Can you work these out from the model? Positions are in its coordinate system, mm. Face numbers are marked on the shaded views. Round coordinates to 2 decimals unless told otherwise and drop trailing zeros. Loops run counter-clockwise (first coordinate to the right, second up) from the corner with the lowest first, then second, coordinate; pieces in that order, holes last. Notation, with made-up numbers: (34.25, 34.5) -> (78.25, 34.5) arc R21 ccw to (78.25, 38.5) -> close; hole circle Ø9 at (37, -29.5). An arc over 180 degrees is marked (long way). Write each question's results on one line, items separated by ' | '.
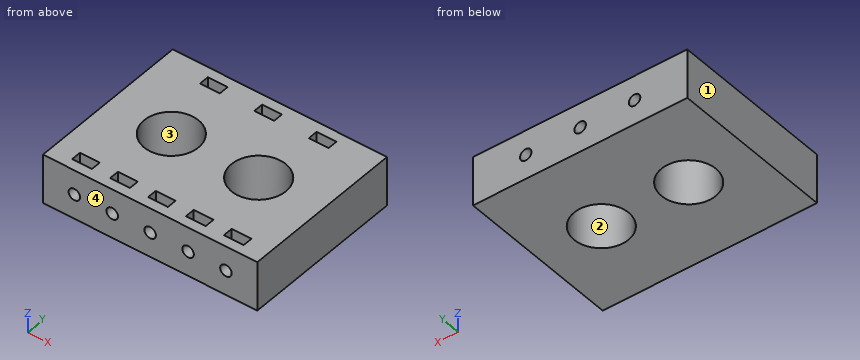
from build123d import *

# Parameters (mm, degrees)
PRISM012_DEPTH            = 3
CYLINDER014_R             = 1.75
CYLINDER014_DEPTH         = 20
BOX014_W                  = 6
BOX014_H                  = 20
BOX014_DEPTH              = 3
FUSION015_PLACEMENT_ANGLE = 180
PRISM013_DEPTH            = 3
CYLINDER015_R             = 1.75
CYLINDER015_DEPTH         = 20
BOX015_W                  = 6
BOX015_H                  = 20
BOX015_DEPTH              = 3
FUSION016_PLACEMENT_ANGLE = 180
PRISM014_DEPTH            = 3
CYLINDER016_R             = 1.75
CYLINDER016_DEPTH         = 20
BOX016_W                  = 6
BOX016_H                  = 20
BOX016_DEPTH              = 3
FUSION017_PLACEMENT_ANGLE = 180
PRISM008_DEPTH            = 3
CYLINDER010_R             = 1.75
CYLINDER010_DEPTH         = 20
BOX010_W                  = 6
BOX010_H                  = 20
BOX010_DEPTH              = 3
PRISM009_DEPTH            = 3
CYLINDER011_R             = 1.75
CYLINDER011_DEPTH         = 20
BOX011_W                  = 6
BOX011_H                  = 20
BOX011_DEPTH              = 3
PRISM010_DEPTH            = 3
CYLINDER012_R             = 1.75
CYLINDER012_DEPTH         = 20
BOX012_W                  = 6
BOX012_H                  = 20
BOX012_DEPTH              = 3
PRISM007_DEPTH            = 3
CYLINDER009_R             = 1.75
CYLINDER009_DEPTH         = 20
BOX009_W                  = 6
BOX009_H                  = 20
BOX009_DEPTH              = 3
PRISM011_DEPTH            = 3
CYLINDER013_R             = 1.75
CYLINDER013_DEPTH         = 20
BOX013_W                  = 6
BOX013_H                  = 20
BOX013_DEPTH              = 3
CYLINDER001_R             = 8.25
CYLINDER001_DEPTH         = 20
CYLINDER_R                = 8.25
CYLINDER_DEPTH            = 20
FUSION_PITCH_ANGLE        = -90
FUSION_PLACEMENT_ANGLE    = 90
BOX_W                     = 65
BOX_H                     = 15
BOX_DEPTH                 = 50
CUT002_PLACEMENT_ANGLE    = 90


with BuildPart() as prisma012:
    # Prism012 → Prism012 (new body)
    with BuildSketch(Plane(origin=(34, 7.5, 3), x_dir=(0, 1, 0), z_dir=(0, 0, 1))):
        Polygon((3.25, 0), (1.625, 2.814583), (-1.625, 2.814583), (-3.25, 0), (-1.625, -2.814583), (1.625, -2.814583), align=None)
    extrude(amount=PRISM012_DEPTH)


with BuildPart() as cilindro014:
    # Cylinder014 → Cylinder014 (new body)
    with BuildSketch(Plane(origin=(34, 7.5, -1), x_dir=(1, 0, 0), z_dir=(0, 0, 1))):
        Circle(CYLINDER014_R)
    extrude(amount=CYLINDER014_DEPTH)


with BuildPart() as fusion015:
    # Box014 → Box014 (new body)
    with BuildSketch(Plane(origin=(31, 9, 3), x_dir=(1, 0, 0), z_dir=(0, 0, 1))):
        with Locations((3, 10)):
            Rectangle(BOX014_W, BOX014_H)
    extrude(amount=BOX014_DEPTH)

    # Fusion015: union Prisma012, Cilindro014
    add(prisma012.part)
    add(cilindro014.part)


with BuildPart() as fusion015_1:
    # Fusion015 placement: moved
    add(fusion015.part.moved(Location((44, 0, 9))).rotate(Axis((44, 0, 9), (0, 1, 0)), FUSION015_PLACEMENT_ANGLE))


with BuildPart() as prisma013:
    # Prism013 → Prism013 (new body)
    with BuildSketch(Plane(origin=(34, 7.5, 3), x_dir=(0, 1, 0), z_dir=(0, 0, 1))):
        Polygon((3.25, 0), (1.625, 2.814583), (-1.625, 2.814583), (-3.25, 0), (-1.625, -2.814583), (1.625, -2.814583), align=None)
    extrude(amount=PRISM013_DEPTH)


with BuildPart() as cilindro015:
    # Cylinder015 → Cylinder015 (new body)
    with BuildSketch(Plane(origin=(34, 7.5, -1), x_dir=(1, 0, 0), z_dir=(0, 0, 1))):
        Circle(CYLINDER015_R)
    extrude(amount=CYLINDER015_DEPTH)


with BuildPart() as fusion016:
    # Box015 → Box015 (new body)
    with BuildSketch(Plane(origin=(31, 9, 3), x_dir=(1, 0, 0), z_dir=(0, 0, 1))):
        with Locations((3, 10)):
            Rectangle(BOX015_W, BOX015_H)
    extrude(amount=BOX015_DEPTH)

    # Fusion016: union Prisma013, Cilindro015
    add(prisma013.part)
    add(cilindro015.part)


with BuildPart() as fusion016_1:
    # Fusion016 placement: moved
    add(fusion016.part.moved(Location((60.5, 0, 9))).rotate(Axis((60.5, 0, 9), (0, 1, 0)), FUSION016_PLACEMENT_ANGLE))


with BuildPart() as prisma014:
    # Prism014 → Prism014 (new body)
    with BuildSketch(Plane(origin=(34, 7.5, 3), x_dir=(0, 1, 0), z_dir=(0, 0, 1))):
        Polygon((3.25, 0), (1.625, 2.814583), (-1.625, 2.814583), (-3.25, 0), (-1.625, -2.814583), (1.625, -2.814583), align=None)
    extrude(amount=PRISM014_DEPTH)


with BuildPart() as cilindro016:
    # Cylinder016 → Cylinder016 (new body)
    with BuildSketch(Plane(origin=(34, 7.5, -1), x_dir=(1, 0, 0), z_dir=(0, 0, 1))):
        Circle(CYLINDER016_R)
    extrude(amount=CYLINDER016_DEPTH)


with BuildPart() as fusion018:
    # Box016 → Box016 (new body)
    with BuildSketch(Plane(origin=(31, 9, 3), x_dir=(1, 0, 0), z_dir=(0, 0, 1))):
        with Locations((3, 10)):
            Rectangle(BOX016_W, BOX016_H)
    extrude(amount=BOX016_DEPTH)

    # Fusion017: union Prisma014, Cilindro016
    add(prisma014.part)
    add(cilindro016.part)


with BuildPart() as fusion018_1:
    # Fusion017 placement: moved
    add(fusion018.part.moved(Location((77, 0, 9))).rotate(Axis((77, 0, 9), (0, 1, 0)), FUSION017_PLACEMENT_ANGLE))

    # Fusion018: union Fusion015, Fusion016
    add(fusion015_1.part)
    add(fusion016_1.part)


with BuildPart() as fusion018_2:
    # Fusion018 placement: moved
    add(fusion018_1.part.moved(Location((6, 0, 0))))


with BuildPart() as prisma008:
    # Prism008 → Prism008 (new body)
    with BuildSketch(Plane(origin=(34, 7.5, 3), x_dir=(0, 1, 0), z_dir=(0, 0, 1))):
        Polygon((3.25, 0), (1.625, 2.814583), (-1.625, 2.814583), (-3.25, 0), (-1.625, -2.814583), (1.625, -2.814583), align=None)
    extrude(amount=PRISM008_DEPTH)


with BuildPart() as cilindro010:
    # Cylinder010 → Cylinder010 (new body)
    with BuildSketch(Plane(origin=(34, 7.5, -1), x_dir=(1, 0, 0), z_dir=(0, 0, 1))):
        Circle(CYLINDER010_R)
    extrude(amount=CYLINDER010_DEPTH)


with BuildPart() as fusion010:
    # Box010 → Box010 (new body)
    with BuildSketch(Plane(origin=(31, 9, 3), x_dir=(1, 0, 0), z_dir=(0, 0, 1))):
        with Locations((3, 10)):
            Rectangle(BOX010_W, BOX010_H)
    extrude(amount=BOX010_DEPTH)

    # Fusion010: union Prisma008, Cilindro010
    add(prisma008.part)
    add(cilindro010.part)


with BuildPart() as fusion010_1:
    # Fusion010 placement: moved
    add(fusion010.part.moved(Location((-9.5, 0, 41))))


with BuildPart() as prisma009:
    # Prism009 → Prism009 (new body)
    with BuildSketch(Plane(origin=(34, 7.5, 3), x_dir=(0, 1, 0), z_dir=(0, 0, 1))):
        Polygon((3.25, 0), (1.625, 2.814583), (-1.625, 2.814583), (-3.25, 0), (-1.625, -2.814583), (1.625, -2.814583), align=None)
    extrude(amount=PRISM009_DEPTH)


with BuildPart() as cilindro011:
    # Cylinder011 → Cylinder011 (new body)
    with BuildSketch(Plane(origin=(34, 7.5, -1), x_dir=(1, 0, 0), z_dir=(0, 0, 1))):
        Circle(CYLINDER011_R)
    extrude(amount=CYLINDER011_DEPTH)


with BuildPart() as fusion011:
    # Box011 → Box011 (new body)
    with BuildSketch(Plane(origin=(31, 9, 3), x_dir=(1, 0, 0), z_dir=(0, 0, 1))):
        with Locations((3, 10)):
            Rectangle(BOX011_W, BOX011_H)
    extrude(amount=BOX011_DEPTH)

    # Fusion011: union Prisma009, Cilindro011
    add(prisma009.part)
    add(cilindro011.part)


with BuildPart() as fusion011_1:
    # Fusion011 placement: moved
    add(fusion011.part.moved(Location((2, 0, 41))))


with BuildPart() as prisma010:
    # Prism010 → Prism010 (new body)
    with BuildSketch(Plane(origin=(34, 7.5, 3), x_dir=(0, 1, 0), z_dir=(0, 0, 1))):
        Polygon((3.25, 0), (1.625, 2.814583), (-1.625, 2.814583), (-3.25, 0), (-1.625, -2.814583), (1.625, -2.814583), align=None)
    extrude(amount=PRISM010_DEPTH)


with BuildPart() as cilindro012:
    # Cylinder012 → Cylinder012 (new body)
    with BuildSketch(Plane(origin=(34, 7.5, -1), x_dir=(1, 0, 0), z_dir=(0, 0, 1))):
        Circle(CYLINDER012_R)
    extrude(amount=CYLINDER012_DEPTH)


with BuildPart() as fusion012:
    # Box012 → Box012 (new body)
    with BuildSketch(Plane(origin=(31, 9, 3), x_dir=(1, 0, 0), z_dir=(0, 0, 1))):
        with Locations((3, 10)):
            Rectangle(BOX012_W, BOX012_H)
    extrude(amount=BOX012_DEPTH)

    # Fusion012: union Prisma010, Cilindro012
    add(prisma010.part)
    add(cilindro012.part)


with BuildPart() as fusion012_1:
    # Fusion012 placement: moved
    add(fusion012.part.moved(Location((13.5, 0, 41))))


with BuildPart() as prisma007:
    # Prism007 → Prism007 (new body)
    with BuildSketch(Plane(origin=(34, 7.5, 3), x_dir=(0, 1, 0), z_dir=(0, 0, 1))):
        Polygon((3.25, 0), (1.625, 2.814583), (-1.625, 2.814583), (-3.25, 0), (-1.625, -2.814583), (1.625, -2.814583), align=None)
    extrude(amount=PRISM007_DEPTH)


with BuildPart() as cilindro009:
    # Cylinder009 → Cylinder009 (new body)
    with BuildSketch(Plane(origin=(34, 7.5, -1), x_dir=(1, 0, 0), z_dir=(0, 0, 1))):
        Circle(CYLINDER009_R)
    extrude(amount=CYLINDER009_DEPTH)


with BuildPart() as fusion009:
    # Box009 → Box009 (new body)
    with BuildSketch(Plane(origin=(31, 9, 3), x_dir=(1, 0, 0), z_dir=(0, 0, 1))):
        with Locations((3, 10)):
            Rectangle(BOX009_W, BOX009_H)
    extrude(amount=BOX009_DEPTH)

    # Fusion009: union Prisma007, Cilindro009
    add(prisma007.part)
    add(cilindro009.part)


with BuildPart() as fusion009_1:
    # Fusion009 placement: moved
    add(fusion009.part.moved(Location((-21, 0, 41))))


with BuildPart() as prisma011:
    # Prism011 → Prism011 (new body)
    with BuildSketch(Plane(origin=(34, 7.5, 3), x_dir=(0, 1, 0), z_dir=(0, 0, 1))):
        Polygon((3.25, 0), (1.625, 2.814583), (-1.625, 2.814583), (-3.25, 0), (-1.625, -2.814583), (1.625, -2.814583), align=None)
    extrude(amount=PRISM011_DEPTH)


with BuildPart() as cilindro013:
    # Cylinder013 → Cylinder013 (new body)
    with BuildSketch(Plane(origin=(34, 7.5, -1), x_dir=(1, 0, 0), z_dir=(0, 0, 1))):
        Circle(CYLINDER013_R)
    extrude(amount=CYLINDER013_DEPTH)


with BuildPart() as fusion014:
    # Box013 → Box013 (new body)
    with BuildSketch(Plane(origin=(31, 9, 3), x_dir=(1, 0, 0), z_dir=(0, 0, 1))):
        with Locations((3, 10)):
            Rectangle(BOX013_W, BOX013_H)
    extrude(amount=BOX013_DEPTH)

    # Fusion013: union Prisma011, Cilindro013
    add(prisma011.part)
    add(cilindro013.part)


with BuildPart() as fusion014_1:
    # Fusion013 placement: moved
    add(fusion014.part.moved(Location((25, 0, 41))))

    # Fusion014: union Fusion010, Fusion011, Fusion012, Fusion009
    add(fusion010_1.part)
    add(fusion011_1.part)
    add(fusion012_1.part)
    add(fusion009_1.part)


with BuildPart() as fusion014_2:
    # Fusion014 placement: moved
    add(fusion014_1.part.moved(Location((-3.5, 0, 0))))


with BuildPart() as cilindro001:
    # Cylinder001 → Cylinder001 (new body)
    with BuildSketch(Plane(origin=(10, 36.5, 0), x_dir=(1, 0, 0), z_dir=(0, 0, 1))):
        Circle(CYLINDER001_R)
    extrude(amount=CYLINDER001_DEPTH)


with BuildPart() as fusion:
    # Cylinder → Cylinder (new body)
    with BuildSketch(Plane(origin=(10, 10, 0), x_dir=(1, 0, 0), z_dir=(0, 0, 1))):
        Circle(CYLINDER_R)
    extrude(amount=CYLINDER_DEPTH)

    # Fusion: union Cilindro001
    add(cilindro001.part)


with BuildPart() as fusion_1:
    # Fusion pitch: moved
    add(fusion.part.rotate(Axis((0, 0, 0), (0, 1, 0)), FUSION_PITCH_ANGLE))


with BuildPart() as fusion_2:
    # Fusion placement: moved
    add(fusion_1.part.moved(Location((55.75, 17, 15))).rotate(Axis((55.75, 17, 15), (0, 0, 1)), FUSION_PLACEMENT_ANGLE))


with BuildPart() as cut002:
    # Box → Box (new body)
    with BuildSketch(Plane.XY):
        with Locations((32.5, 7.5)):
            Rectangle(BOX_W, BOX_H)
    extrude(amount=BOX_DEPTH)

    # Cut: cut Fusion
    add(fusion_2.part, mode=Mode.SUBTRACT)

    # Cut001: cut Fusion014
    add(fusion014_2.part, mode=Mode.SUBTRACT)

    # Cut002: cut Fusion018
    add(fusion018_2.part, mode=Mode.SUBTRACT)


with BuildPart() as cut002_1:
    # Cut002 placement: moved
    add(cut002.part.rotate(Axis((0, 0, 0), (1, 0, 0)), CUT002_PLACEMENT_ANGLE))


solid = cut002_1.part
1. Please list where these lines run through material, in increasing order: line 1 (X direction, y = -25, z = 7.5); line 2 (X direction, y = -17.5, z = 9.5); line 3 (Y direction, x = 18.5, z = 9.5). Write a range as from..to.
Final values:
line 1: 0..11, 27.5..37.5, 54..65 | line 2: 0..15.81, 22.69..42.31, 49.19..65 | line 3: -50..-47, -44..-33.22, -16.78..-6, -3..0
2. If we section it at C-C (y = -8): List the corners of the cut face in (x, z) for me.
Final values:
outline: (0, 0) -> (65, 0) -> (65, 15) -> (0, 15) -> close; hole circle Ø3.5 at (16, 7.5); hole circle Ø3.5 at (32.5, 7.5); hole circle Ø3.5 at (49, 7.5)
3. If we section it at D-D (z = 12.5): State how many separate pieces and enclosed holes the cut face has, then the cut area to 3 significant figures.
Final values:
separate pieces: 1 | enclosed holes: 10 | area: 2,680 mm2
4. We'd pull the mould along X, two halves only. Please class the marked faces 1, 2, 3 and 4: pulls with the +X half, pulls with the -X half, needs draft (parallel to the pull), parting line crosses it, or undercut.
Final values:
face 1: pulls with the -X half | face 2: undercut | face 3: undercut | face 4: needs draft
5. If we section it at B-B (z = 3.5): List the corners of the cut face in (x, y) for me.
Final values:
outline: (0, -50) -> (65, -50) -> (65, 0) -> (0, 0) -> close; hole circle Ø16.5 at (19.25, -25); hole circle Ø16.5 at (45.75, -25)
6. Will this pin go through, and if not, where does the flat tip stop? pin 1 (4.5 mm diameter, centred on x = 16, z = 7.5, fed in from +Y).
Final values:
pin 1: y = 0
7. If we section it at A-A (y = -25): List the corners of the cut face in (x, z) for me.
Final values:
outline: (0, 0) -> (11, 0) -> (11, 15) -> (0, 15) -> close; (27.5, 0) -> (37.5, 0) -> (37.5, 15) -> (27.5, 15) -> close; (54, 0) -> (65, 0) -> (65, 15) -> (54, 15) -> close
